```python
from build123d import *

# Parameters (mm, degrees)
SKETCH1_W            = 40
SKETCH1_H            = 50
BOSS_EXTRUDE1_DEPTH  = 5
SKETCH4_W            = 5
SKETCH4_H            = 5
BOSS_EXTRUDE4_DEPTH  = 20
SKETCH4_4_W          = 15
SKETCH4_4_H          = 5
BOSS_EXTRUDE5_DEPTH  = 10
CUT_EXTRUDE2_DEPTH   = 4
BOSS_EXTRUDE7_START  = 3
BOSS_EXTRUDE7_DEPTH  = 3
SKETCH11_W           = 5
SKETCH11_H           = 5
BOSS_EXTRUDE8_DEPTH  = 5
SKETCH12_R           = 1.5
CUT_EXTRUDE6_DEPTH   = 5
SKETCH15_W           = 5
SKETCH15_H           = 2.5
BOSS_EXTRUDE11_DEPTH = 5
BOSS_EXTRUDE12_DEPTH = 10
SKETCH16_R           = 1.5
CUT_EXTRUDE8_DEPTH   = 2.5
SKETCH18_R           = 1.05
CUT_EXTRUDE9_DEPTH   = 5


with BuildPart() as part:
    # Sketch1 → Boss-Extrude1 (new body)
    with BuildSketch(Plane(origin=(0, 0, 0), x_dir=(1, 0, 0), z_dir=(0, 1, 0))):
        Rectangle(SKETCH1_W, SKETCH1_H)
    extrude(amount=BOSS_EXTRUDE1_DEPTH)

    # Sketch4 → Boss-Extrude4 (add)
    with BuildSketch(Plane(origin=(0, 5, 0), x_dir=(1, 0, 0), z_dir=(0, 1, 0))):
        with Locations((-9.5, -22.5)):
            Rectangle(SKETCH4_W, SKETCH4_H)
        with Locations((-17.5, 22.5)):
            Rectangle(SKETCH4_W, SKETCH4_H)
    extrude(amount=BOSS_EXTRUDE4_DEPTH)

    # Sketch4_4 → Boss-Extrude5 (add)
    with BuildSketch(Plane(origin=(0, 5, 0), x_dir=(1, 0, 0), z_dir=(0, 1, 0))):
        Polygon((20, -25), (20, 25), (16, 25), (16, -20), (-7, -20), (-7, -25), align=None)
        with Locations((0.5, 22.5)):
            Rectangle(SKETCH4_4_W, SKETCH4_4_H)
    extrude(amount=BOSS_EXTRUDE5_DEPTH)

    # Sketch7 → Cut-Extrude2 (cut)
    with BuildSketch(Plane(origin=(20, 0, 0), x_dir=(0, 0, -1), z_dir=(1, 0, 0))):
        with BuildLine():
            Line((-1, 15), (21, 15))
            ThreePointArc((21, 15), (10, 4), (-1, 15))
        make_face()
    extrude(amount=-CUT_EXTRUDE2_DEPTH, mode=Mode.SUBTRACT)

    # Sketch8 → Boss-Extrude7 (add)
    with BuildSketch(Plane(origin=(20, 0, 0), x_dir=(0, 0, -1), z_dir=(1, 0, 0)).offset(BOSS_EXTRUDE7_START)):
        with BuildLine():
            Line((-1, 15), (-4, 15))
            Line((-4, 15), (-4, 0))
            Line((-4, 0), (24, 0))
            Line((24, 0), (24, 15))
            Line((24, 15), (21, 15))
            ThreePointArc((21, 15), (10, 4), (-1, 15))
        make_face()
    extrude(amount=-BOSS_EXTRUDE7_DEPTH)

    # Sketch11 → Boss-Extrude8 (add)
    with BuildSketch(Plane(origin=(0, 0, -25), x_dir=(-1, 0, 0), z_dir=(0, 0, -1))):
        with Locations((0, 12.5)):
            Rectangle(SKETCH11_W, SKETCH11_H)
    extrude(amount=BOSS_EXTRUDE8_DEPTH)

    # Sketch12 → Cut-Extrude6 (cut)
    with BuildSketch(Plane.XZ.offset(-10)):
        with Locations(Location((0, -27.5, 0), (0, 0, 270))):
            Circle(SKETCH12_R)
    extrude(amount=-CUT_EXTRUDE6_DEPTH, mode=Mode.SUBTRACT)

    # Sketch15 → Boss-Extrude11 (add)
    with BuildSketch(Plane.XY.offset(25)):
        with Locations((10, 11.25)):
            Rectangle(SKETCH15_W, SKETCH15_H)
    extrude(amount=BOSS_EXTRUDE11_DEPTH)

    # Sketch15_3 → Boss-Extrude12 (add)
    with BuildSketch(Plane.XY.offset(25)):
        Polygon((7.5, 10), (7.5, 12.5), (-7.5, 12.5), (-7.5, 5), (7.5, 5), align=None)
    extrude(amount=BOSS_EXTRUDE12_DEPTH)

    # Sketch16 → Cut-Extrude8 (cut)
    with BuildSketch(Plane.XZ.offset(-10)):
        with Locations((10, 27.5)):
            Circle(SKETCH16_R)
    extrude(amount=-CUT_EXTRUDE8_DEPTH, mode=Mode.SUBTRACT)

    # Sketch18 → Cut-Extrude9 (cut)
    with BuildSketch(Plane.XZ):
        with Locations(Location((-7, 7, 0), (0, 0, 270))):
            Circle(SKETCH18_R)
        with Locations(Location((7, 7, 0), (0, 0, 90))):
            Circle(SKETCH18_R)
        with Locations(Location((7, -7, 0), (0, 0, 270))):
            Circle(SKETCH18_R)
        with Locations(Location((-7, -7, 0), (0, 0, 90))):
            Circle(SKETCH18_R)
    extrude(amount=-CUT_EXTRUDE9_DEPTH, mode=Mode.SUBTRACT)


solid = part.part
```
Read the model definition and answer for the solid it produces. Units are mm, in the model's axes. A direction names the side the tool comes from. Coordinates: 2 decimals unless noted, no trailing zeros. Write each loop counter-clockwise with the first axis right and the second up, starting at its lowest first coordinate (ties: lowest second). Pieces come first, ordered by that corner, then holes. Notation, with made-up numbers: (-27.75, 82.5) -> (26.25, 82.5) arc R7 ccw to (26.25, 92.5) -> close; hole circle Ø2 at (67, 23.5). An arc over 180 degrees is marked (long way). Write item = value, one per line.
(1) Given pin 1 Ø5 at (x, y) = (17, 10) entering from -Z; pin 2 Ø4 at (x, z) = (-7.5, -13.5) entering from +Y; pin 3 Ø2 at (y, z) = (7.5, 31) entering from +X, each flat-ended and moving along its own axis, determine where each tip first touches the part or whether it passes through.
From the geometry:
pin_1 = -25
pin_2 = 5
pin_3 = 7.5
(2) Section D-D on z = -10 is taken. Write down the section's boundary in (x, y), plus the area to 3 significant figures.
From the geometry:
outline = (-20, 0) -> (23, 0) -> (23, 4) -> (16, 4) -> (16, 5) -> (-20, 5) -> close
area = 208 mm2
(3) Which of the six approach directions +Z, -Z, +X, -X, +Y, -Y give full straight-line access (tool end or side, diameter ignored) to faces 1 (the face through (22, 7, -24)), 2 (the face through (-18, 15, -20)), 3 (the face through (-7, 10, -22)), 4 (the face through (0, 10, -20))?
From the geometry:
face_1 = -Z, +X, +Y, -Y
face_2 = +Z, -X, +Y
face_3 = -Z, +Y
face_4 = -X, +Y
(4) Section A-A on x = 10 is taken. Write down the section's boundary in (y, z).
From the geometry:
outline = (0, -25) -> (5, -25) -> (5, 20) -> (15, 20) -> (15, 25) -> (12.5, 25) -> (12.5, 26) -> (10, 26) -> (10, 25) -> (0, 25) -> close; (10, 29) -> (12.5, 29) -> (12.5, 30) -> (10, 30) -> close
(5) Section B-B on y = 15.75 is taken. Write down the section's boundary in (x, z), plus the area to 3 significant figures.
From the geometry:
outline = (-20, -25) -> (-15, -25) -> (-15, -20) -> (-20, -20) -> close; (-12, 20) -> (-7, 20) -> (-7, 25) -> (-12, 25) -> close
area = 50.0 mm2
(6) Section C-C on z = 27.5 is taken. Write down the section's boundary in (x, y), plus the area to 4 significant figures.
From the geometry:
outline = (-7.5, 5) -> (7.5, 5) -> (7.5, 10) -> (8.5, 10) -> (8.5, 12.5) -> (-7.5, 12.5) -> close; (11.5, 10) -> (12.5, 10) -> (12.5, 12.5) -> (11.5, 12.5) -> close
area = 117.5 mm2
(7) For a pull along X with two mould halves and no side action, classify faces 5 (the face through (-7, 20, 23)), 6 (the face through (-2.5, 12, -27)), 7 (the face through (2, 0, 0)), 8 (the face through (-7.05, 2.46, -8.05)) as +X half, -X half, draft (parallel to the pull), parting line (faces both ways), or undercut.
From the geometry:
face_5 = +X half
face_6 = -X half
face_7 = draft
face_8 = undercut
(8) Straight lines are drawn through the part: L1, parallel to X at y = 2.6, z = 7; L2, parallel to X at y = 2.75, z = -7; L3, parallel to X at y = 12.3, z = -27.5. For each, find the intervals that lie inside material, in ascending order. Write a range as from..to.
From the geometry:
L1 = -20..-8.05, -5.95..5.95, 8.05..20
L2 = -20..-8.05, -5.95..5.95, 8.05..23
L3 = -2.5..-1.5, 1.5..2.5
